CAD build for the part. Positions are in the model's coordinates, mm. A direction names the side the tool comes from. Coordinates: 2 decimals unless noted, no trailing zeros. Order: outer loops, then holes, each group sorted by start corner. A loop starts at its lowest first (then second) coordinate and runs counter-clockwise, first axis right, second up. Notation, with made-up numbers: M 38.25,58 L 55.25,58 A29 cw 55.25,79 Z; hole C 42.5,82.25 d3. An arc over 180 degrees is marked long. Write item = value, one per line.
from build123d import *

# Parameters (mm, degrees)
SKETCH1_W           = 300
SKETCH1_H           = 300
SKETCH1_W_2         = 287.3
SKETCH1_H_2         = 287.3
BOSS_EXTRUDE1_DEPTH = 39.8272
CUT_EXTRUDE1_REACH  = 339.766
SKETCH3_W           = 15.3
SKETCH3_H           = 12.7
SKETCH3_W_2         = 9
SKETCH3_H_2         = 11


with BuildPart() as part:
    # Sketch1 → Boss-Extrude1 (new body)
    with BuildSketch(Plane(origin=(0, 0, 0), x_dir=(1, 0, 0), z_dir=(0, 1, 0))):
        Rectangle(SKETCH1_W, SKETCH1_H)
        Rectangle(SKETCH1_W_2, SKETCH1_H_2, mode=Mode.SUBTRACT)
    extrude(amount=BOSS_EXTRUDE1_DEPTH)

    # Sketch3 → Cut-Extrude1 (cut, up to next)
    with BuildSketch(Plane(origin=(0, 0, -150), x_dir=(-1, 0, 0), z_dir=(0, 0, -1)), mode=Mode.PRIVATE) as cut_extrude1_sk1:
        Polygon((-72.497624126, 13.305953258), (-72.497624126, 17.418810742), (-107.152019667, 17.418810742), (-107.152019667, 13.305953258), (-105.517624126, 13.305953258), (-105.517624126, 6.4008), (-89.515624126, 6.4008), (-89.515624126, 13.305953258), align=None)
    cut_extrude1_tool1 = extrude(cut_extrude1_sk1.sketch, amount=-CUT_EXTRUDE1_REACH, mode=Mode.PRIVATE) & part.part
    # Sketch3 → Cut-Extrude1 (cut, up to next)
    with BuildSketch(Plane(origin=(0, 0, -150), x_dir=(-1, 0, 0), z_dir=(0, 0, -1)), mode=Mode.PRIVATE) as cut_extrude1_sk2:
        with Locations((-38.618448478, 7.9248)):
            Rectangle(SKETCH3_W, SKETCH3_H)
    cut_extrude1_tool2 = extrude(cut_extrude1_sk2.sketch, amount=-CUT_EXTRUDE1_REACH, mode=Mode.PRIVATE) & part.part
    # Sketch3 → Cut-Extrude1 (cut, up to next)
    with BuildSketch(Plane(origin=(0, 0, -150), x_dir=(-1, 0, 0), z_dir=(0, 0, -1)), mode=Mode.PRIVATE) as cut_extrude1_sk3:
        with Locations((-18.092571078, 7.9248)):
            Rectangle(SKETCH3_W, SKETCH3_H)
    cut_extrude1_tool3 = extrude(cut_extrude1_sk3.sketch, amount=-CUT_EXTRUDE1_REACH, mode=Mode.PRIVATE) & part.part
    # Sketch3 → Cut-Extrude1 (cut, up to next)
    with BuildSketch(Plane(origin=(0, 0, -150), x_dir=(-1, 0, 0), z_dir=(0, 0, -1)), mode=Mode.PRIVATE) as cut_extrude1_sk4:
        with Locations((6.757428922, 7.1748)):
            Rectangle(SKETCH3_W_2, SKETCH3_H_2)
    cut_extrude1_tool4 = extrude(cut_extrude1_sk4.sketch, amount=-CUT_EXTRUDE1_REACH, mode=Mode.PRIVATE) & part.part
    # Sketch3 → Cut-Extrude1 (cut, up to next)
    with BuildSketch(Plane(origin=(0, 0, -150), x_dir=(-1, 0, 0), z_dir=(0, 0, -1)), mode=Mode.PRIVATE) as cut_extrude1_sk5:
        with Locations((28.457428922, 7.1748)):
            Rectangle(SKETCH3_W_2, SKETCH3_H_2)
    cut_extrude1_tool5 = extrude(cut_extrude1_sk5.sketch, amount=-CUT_EXTRUDE1_REACH, mode=Mode.PRIVATE) & part.part
    add(cut_extrude1_tool1.solids().sort_by_distance((93.183841, 12.956593, -150))[0], mode=Mode.SUBTRACT)
    add(cut_extrude1_tool2.solids().sort_by_distance((38.618448, 7.9248, -150))[0], mode=Mode.SUBTRACT)
    add(cut_extrude1_tool3.solids().sort_by_distance((18.092571, 7.9248, -150))[0], mode=Mode.SUBTRACT)
    add(cut_extrude1_tool4.solids().sort_by_distance((-6.757429, 7.1748, -150))[0], mode=Mode.SUBTRACT)
    add(cut_extrude1_tool5.solids().sort_by_distance((-28.457429, 7.1748, -150))[0], mode=Mode.SUBTRACT)


solid = part.part
(1) Pin check, flat tip, straight feed: pin 1 Ø7 at (x, z) = (86.5, -146.5) entering from -Y. Stop position of the tip, or through.
Evaluation:
pin_1 = 0
(2) Slice it at A-A, the plane x = 83.5. Write the cut outline in (y, z).
Evaluation:
outline = M 0,-150 L 13.31,-150 L 13.31,-143.65 L 0,-143.65 Z; M 0,143.65 L 39.83,143.65 L 39.83,150 L 0,150 Z; M 17.42,-150 L 39.83,-150 L 39.83,-143.65 L 17.42,-143.65 Z
(3) Slice it at C-C, the plane x = -66. Write the cut outline in (y, z), then the cut area to 3 significant figures.
Evaluation:
outline = M 0,-150 L 39.83,-150 L 39.83,-143.65 L 0,-143.65 Z; M 0,143.65 L 39.83,143.65 L 39.83,150 L 0,150 Z
area = 506 mm²
(4) Slice it at D-D, the plane z = -122.5. Write the cut outline in (x, y), then the cut area to 3 significant figures.
Evaluation:
outline = M -150,0 L -143.65,0 L -143.65,39.83 L -150,39.83 Z; M 143.65,0 L 150,0 L 150,39.83 L 143.65,39.83 Z
area = 506 mm²
(5) Tool access for faces 1 (the face through (-143.65, 20, 2)), 2 (the face through (-12, 0, 144)): list every direction of +Z, -Z, +X, -X, +Y, -Y with a clear straight run to the whole face (end or side of a thin tool).
Evaluation:
face_1 = +Y, -Y
face_2 = +Z, -Z, +X, -X, -Y
(6) Pull direction X, two halves, no side cores. Call faces 3 (the face through (-150, 20, 2)), 4 (the face through (-12, 39.827, 144)), 5 (the face through (-2, 20, -143.65)): +X half, -X half, draft (parallel to the pull), parting line (faces both ways), or undercut.
Evaluation:
face_3 = -X half
face_4 = draft
face_5 = undercut
(7) Wall check: line 1 (Z direction, x = 131.5, y = 28); line 2 (Z direction, x = -9, y = 4). Give the ranges that are in metal, low to high. Write a range as from..to.
Evaluation:
line_1 = -150..-143.65, 143.65..150
line_2 = 143.65..150
(8) Slice it at B-B, the plane y = 35. Write the cut outline in (x, z), then the cut area to 3 significant figures.
Evaluation:
outline = M -150,-150 L 150,-150 L 150,150 L -150,150 Z; hole M -143.65,-143.65 L 143.65,-143.65 L 143.65,143.65 L -143.65,143.65 Z
area = 7,460 mm²
